Design review of the part built by this model. Coordinates are the model's own, in mm. A direction names the side the tool comes from. Give positions to 0.01 mm unless a question says otherwise; leave off trailing zeros. Write each loop counter-clockwise with the first axis right and the second up, starting at its lowest first coordinate (ties: lowest second). Pieces come first, ordered by that corner, then holes.
```python
from build123d import *

# Parameters (mm, degrees)
F0_W     = 60
F0_H     = 125
F1_DEPTH = 55
F2_W     = 54
F2_H     = 105
F3_DEPTH = 55.001
F4_R     = 7.978421
F5_DEPTH = 55.001
F6_W     = 47.78267
F6_H     = 39
F7_DEPTH = 125.001
F8_W     = 35
F8_H     = 105
F9_DEPTH = 6.001


with BuildPart() as f1:
    # F0 (on Front) → F1 (new body)
    with BuildSketch(Plane.XZ):
        with Locations((-9.565847, 0)):
            Rectangle(F0_W, F0_H)
    extrude(amount=F1_DEPTH)

    # F2 (on face) → F3 (cut, through all)
    with BuildSketch(Plane.XZ.offset(55)):
        with Locations((-12.565847, 0)):
            Rectangle(F2_W, F2_H)
    extrude(amount=-F3_DEPTH, mode=Mode.SUBTRACT)

    # F4 (on face) → F5 (cut, through all)
    with BuildSketch(Plane.XZ.offset(55)):
        with Locations((-39.565847, 57.5)):
            Circle(F4_R)
        with Locations((-39.565847, -57.5)):
            Circle(F4_R)
    extrude(amount=-F5_DEPTH, mode=Mode.SUBTRACT)

    # F6 (on face) → F7 (cut, through all)
    with BuildSketch(Plane.XY.offset(62.5)):
        with Locations((-9.457182, -27.5)):
            Rectangle(F6_W, F6_H)
    extrude(amount=-F7_DEPTH, mode=Mode.SUBTRACT)

    # F8 (on face) → F9 (cut, through all)
    with BuildSketch(Plane(origin=(14.434153, 0, 0), x_dir=(0, -1, 0), z_dir=(-1, 0, 0))):
        with Locations((27.5, 0)):
            Rectangle(F8_W, F8_H)
    extrude(amount=-F9_DEPTH, mode=Mode.SUBTRACT)


solid = f1.part
```
(1) Tool access review of faces 1 (the face through (-10, -4, 52.5)), 2 (the face through (-10, -47, 58)), 3 (the face through (15, -29, 62.5)), 4 (the face through (17, -45, -1)): name each direction out of +Z, -Z, +X, -X, +Y, -Y from which nothing blocks a thin tool from reaching the whole face with its end or side.
Resolved:
face 1: -X, +Y, -Y
face 2: +Z, -Z, -X
face 3: +Z, +X, -X, +Y, -Y
face 4: +X, -X
(2) Clearance check with a flat-ended pin moving along its axis: P1, Ø8, axis at x = 1, z = 57.5, coming from the +Y side. State where the tip first meets the part, or that it passes through.
Resolved:
P1: stops at y = 0
(3) Consider section A-A, the plane z = 37. Give the boundary of the cut face in (x, y).
Resolved:
outline: (14.43, -55) - (20.43, -55) - (20.43, -45) - (14.43, -45) - close; (14.43, -10) - (20.43, -10) - (20.43, 0) - (14.43, 0) - close
(4) To check wall thickness, follow L1, parallel to Y at x = 16.5, z = -40.5; L2, parallel to Z at x = 17, y = -27; L3, parallel to X at y = -9, z = -55.5. State the ranges of each line that lie inside material, in increasing order.
Resolved:
L1: y = -55 to -45, -10 to 0
L2: z = -62.5 to -52.5, 52.5 to 62.5
L3: x = 14.43 to 20.43
(5) Consider section C-C, the plane y = -34. Give the boundary of the cut face in (x, z), then the cut area to 3 significant figures.
Resolved:
outline: (14.43, -62.5) - (20.43, -62.5) - (20.43, -52.5) - (14.43, -52.5) - close; (14.43, 52.5) - (20.43, 52.5) - (20.43, 62.5) - (14.43, 62.5) - close
area: 120 mm2
(6) Mouldability with a two-part tool opening along Z and no side actions: class faces 5 (the face through (20.434, -45.4, -0.9)), 6 (the face through (15, -29, -62.5)), 7 (the face through (-31.588, -4.056, -57.576)) as pulls with the +Z half, pulls with the -Z half, needs draft (parallel to the pull), parting line crosses it, or undercut.
Resolved:
face 5: needs draft
face 6: pulls with the -Z half
face 7: undercut
(7) Consider section B-B, the plane x = 13. Give the boundary of the cut face in (y, z).
Resolved:
outline: (-55, -62.5) - (-47, -62.5) - (-47, -52.5) - (-55, -52.5) - close; (-55, 52.5) - (-47, 52.5) - (-47, 62.5) - (-55, 62.5) - close; (-8, -62.5) - (0, -62.5) - (0, -52.5) - (-8, -52.5) - close; (-8, 52.5) - (0, 52.5) - (0, 62.5) - (-8, 62.5) - close
